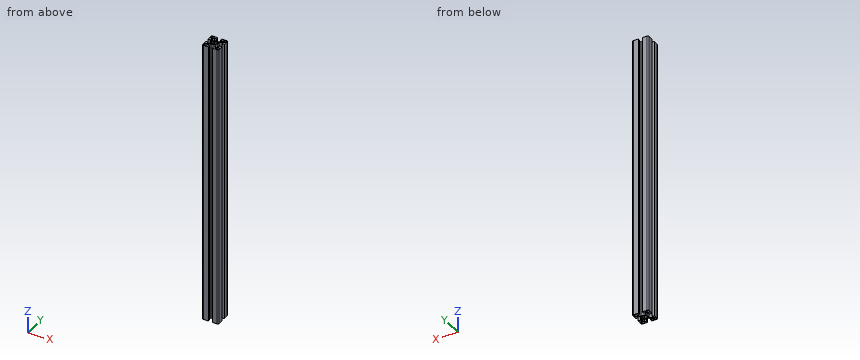
Autodesk Inventor part; units mm, degrees
ref_plane "YZ Plane" through (0, 0, 0) normal (1, 0, 0) x (0, 1, 0)
ref_plane "XZ Plane" through (0, 0, 0) normal (0, 1, 0) x (-1, 0, 0)
ref_plane "XY Plane" through (0, 0, 0) normal (0, 0, 1) x (1, 0, 0)
sketch "T-Slot 4040 Base" plane through (0, 0, 0) normal (0, 0, 1) x (1, 0, 0)
  line L0 (-28, 0) -> (28, 0) construction
  line L1 (0, -28) -> (0, 28) construction
  circle A0 centre (0, 0) radius 5.1
  line L2 (-7.5, -7.5) -> (7.5, -7.5)
  line L3 (7.5, -7.5) -> (7.5, 7.5)
  line L4 (7.5, 7.5) -> (-7.5, 7.5)
  line L5 (-7.5, 7.5) -> (-7.5, -7.5)
  line L6 (-7.5, -7.5) -> (7.5, 7.5) construction
  line L7 (7.5, -7.5) -> (-7.5, 7.5) construction
  line L8 (-20, 20) -> (20, 20)
  line L9 (20, 20) -> (20, -20)
  line L10 (20, -20) -> (-20, -20)
  line L11 (-20, -20) -> (-20, 20)
  line L12 (-20, 20) -> (20, -20) construction
  line L13 (20, 20) -> (-20, -20) construction
  line L14 (20, 5) -> (14.5, 5)
  line L15 (14.5, 5) -> (14.5, 10)
  line L16 (14.5, 10) -> (12.4749, 10)
  line L17 (12.4749, 10) -> (7.5, 5.0251)
  line L18 (5, 20) -> (5, 14.5)
  line L19 (5, 14.5) -> (10, 14.5)
  line L20 (10, 14.5) -> (10, 12.4749)
  line L21 (10, 12.4749) -> (5.0251, 7.5)
  line L22 (18.5, 18.5) -> (11.5, 18.5)
  line L23 (11.5, 18.5) -> (11.5, 11.5)
  line L24 (11.5, 11.5) -> (18.5, 11.5)
  line L25 (18.5, 11.5) -> (18.5, 18.5)
  line L26 (18.5, 18.5) -> (11.5, 11.5) construction
  line L27 (11.5, 18.5) -> (18.5, 11.5) construction
  line L28 (3.0732, 1.3088) -> (4.38, 2.6125) construction
  line L29 (5.905, 4.1338) -> (4.1393, 5.9037)
  line L30 (4.1393, 5.9037) -> (2.6122, 4.3802)
  line L31 (1.3075, 3.0787) -> (3.0732, 1.3088) construction
  line L32 (3.0732, 1.3088) -> (4.1393, 5.9037) construction
  line L33 (5.905, 4.1338) -> (1.3075, 3.0787) construction
  line L34 (4.38, 2.6125) -> (5.905, 4.1338)
  line L35 (2.6122, 4.3802) -> (1.3075, 3.0787) construction
  line L36 (-20, 5) -> (-14.5, 5)
  line L37 (-14.5, 5) -> (-14.5, 10)
  line L38 (-14.5, 10) -> (-12.4749, 10)
  line L39 (-12.4749, 10) -> (-7.5, 5.0251)
  line L40 (-5, 20) -> (-5, 14.5)
  line L41 (-5, 14.5) -> (-10, 14.5)
  line L42 (-10, 14.5) -> (-10, 12.4749)
  line L43 (-10, 12.4749) -> (-5.0251, 7.5)
  line L44 (-18.5, 18.5) -> (-11.5, 18.5)
  line L45 (-11.5, 18.5) -> (-11.5, 11.5)
  line L46 (-11.5, 11.5) -> (-18.5, 11.5)
  line L47 (-18.5, 11.5) -> (-18.5, 18.5)
  line L48 (-5.905, 4.1338) -> (-4.1393, 5.9037)
  line L49 (-4.1393, 5.9037) -> (-2.6122, 4.3802)
  line L50 (-4.38, 2.6125) -> (-5.905, 4.1338)
  line L51 (7.5, -7.5) -> (-7.5, -7.5)
  line L52 (20, -5) -> (14.5, -5)
  line L53 (14.5, -5) -> (14.5, -10)
  line L54 (14.5, -10) -> (12.4749, -10)
  line L55 (12.4749, -10) -> (7.5, -5.0251)
  line L56 (5, -20) -> (5, -14.5)
  line L57 (5, -14.5) -> (10, -14.5)
  line L58 (10, -14.5) -> (10, -12.4749)
  line L59 (10, -12.4749) -> (5.0251, -7.5)
  line L60 (18.5, -18.5) -> (11.5, -18.5)
  line L61 (11.5, -18.5) -> (11.5, -11.5)
  line L62 (11.5, -11.5) -> (18.5, -11.5)
  line L63 (18.5, -11.5) -> (18.5, -18.5)
  line L64 (18.5, -18.5) -> (11.5, -11.5) construction
  line L65 (11.5, -18.5) -> (18.5, -11.5) construction
  line L66 (3.0732, -1.3088) -> (4.38, -2.6125) construction
  line L67 (5.905, -4.1338) -> (4.1393, -5.9037)
  line L68 (4.1393, -5.9037) -> (2.6122, -4.3802)
  line L69 (1.3075, -3.0787) -> (3.0732, -1.3088) construction
  line L70 (3.0732, -1.3088) -> (4.1393, -5.9037) construction
  line L71 (5.905, -4.1338) -> (1.3075, -3.0787) construction
  line L72 (4.38, -2.6125) -> (5.905, -4.1338)
  line L73 (2.6122, -4.3802) -> (1.3075, -3.0787) construction
  line L74 (-4.38, -2.6125) -> (-5.905, -4.1338)
  line L75 (-4.1393, -5.9037) -> (-2.6122, -4.3802)
  line L76 (-5.905, -4.1338) -> (-4.1393, -5.9037)
  line L77 (-12.4749, -10) -> (-7.5, -5.0251)
  line L78 (-10, -12.4749) -> (-5.0251, -7.5)
  line L79 (-10, -14.5) -> (-10, -12.4749)
  line L80 (-5, -14.5) -> (-10, -14.5)
  line L81 (-5, -20) -> (-5, -14.5)
  line L82 (-18.5, -18.5) -> (-11.5, -18.5)
  line L83 (-11.5, -18.5) -> (-11.5, -11.5)
  line L84 (-11.5, -11.5) -> (-18.5, -11.5)
  line L85 (-18.5, -11.5) -> (-18.5, -18.5)
  line L86 (-14.5, -10) -> (-12.4749, -10)
  line L87 (-14.5, -5) -> (-14.5, -10)
  line L88 (-20, -5) -> (-14.5, -5)
  point P0 (15, 15)
  point P1 (3.6062, 3.6062)
  point P2 (3.6062, 3.6062)
  point P3 (15, -15)
  point P4 (3.6062, -3.6062)
  point P5 (3.6062, -3.6062)
  dimension "d9" = 10.2
  dimension "d12" = 40
  dimension "d13" = 40
  dimension "d14" = 5.5
  dimension "d15" = 15
  dimension "d16" = 7
  dimension "d17" = 10
  dimension "d20" = 1.75
  dimension "d21" = 7
  dimension "d22" = 2
  dimension "d29" = 1.5
  dimension "d30" = 2.5
extrude "Extrusion1" add sketch "T-Slot 4040 Base" along normal blind 705 contours L5 L4 L3 L2 | L2 L78 L79 L80 L81 L10 L11 L88 L87 L86 L77 L5 | L2 L3 L55 L54 L53 L52 L9 L10 L56 L57 L58 L59 | L39 L38 L37 L36 L11 L8 L40 L41 L42 L43 L4 L5 | L3 L4 L21 L20 L19 L18 L8 L9 L14 L15 L16 L17
fillet "Rundung1" radius 1 16 edges at (11.5, 18.5, 352.5) (18.5, 18.5, 352.5) (18.5, 11.5, 352.5) (11.5, 11.5, 352.5) (-11.5, 18.5, 352.5) (-18.5, 18.5, 352.5) (-18.5, 11.5, 352.5) (-11.5, 11.5, 352.5) (-18.5, -11.5, 352.5) (-11.5, -11.5, 352.5) (-11.5, -18.5, 352.5) (-18.5, -18.5, 352.5) (11.5, -18.5, 352.5) (11.5, -11.5, 352.5) (18.5, -11.5, 352.5) (18.5, -18.5, 352.5)
fillet "Rundung2" radius 3 4 edges at (20, 20, 352.5) (20, -20, 352.5) (-20, -20, 352.5) (-20, 20, 352.5)
properties part number "T-SLOT 4040 B-Type 705mm"
The model under review builds one solid part; all positions refer to its coordinate system, in mm. Round coordinates to 2 decimals unless told otherwise and drop trailing zeros. Write item = value, one per line. Start each with the question number.
Item 1: To check wall thickness, follow L1, parallel to X at y = -13.5, z = 577; L2, parallel to Y at x = 16, z = 193; L3, parallel to X at y = 4, z = 656. State the ranges of each line that lie inside material, in increasing order.
Item 2: Insertion check: pin 1 (3 mm diameter, centred on x = -0.5, z = 297.5, fed in from -Y); pin 2 (3 mm diameter, centred on y = -0.5, z = 242.5, fed in from +X). Each pin has a flat end and moves straight along its axis. Give the tip position at first contact, or say it passes through.
Item 3: Take a section at A-A on z = 617. Count the separate pieces of the cut face and the enclosed holes in it, plus the area to 3 significant figures.
Result:
q1.L1 = -20 to -18.5, -11.5 to -10, 10 to 11.5, 18.5 to 20
q1.L2 = -20 to -18.5, -11.5 to -5, 5 to 11.5, 18.5 to 20
q1.L3 = -7.5 to -5.77, 5.77 to 7.5
q2.pin_1 = -7.5
q2.pin_2 = 7.5
q3.separate_pieces = 1
q3.enclosed_holes = 5
q3.area = 616 mm²
